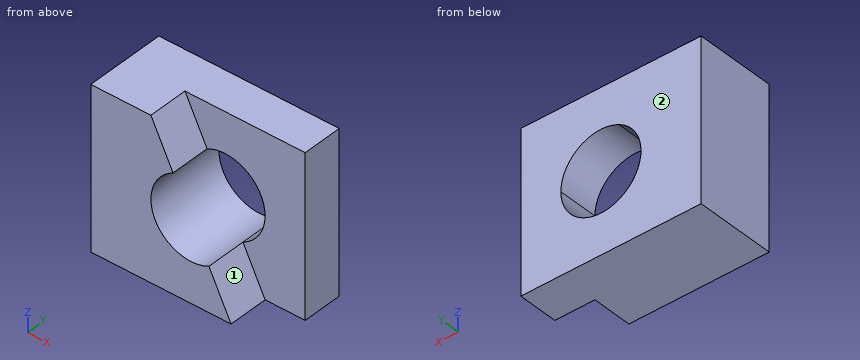
```python
from build123d import *

# Parameters (mm, degrees)
F0_W     = 57.15
F0_H     = 50.8
F1_DEPTH = 25.4
F3_DEPTH = 12.7
F5_DEPTH = 25.4


# Not quite as in the source:
# - a feature of the source that left no trace in its solid (it failed there, or was rolled back) is left out


with BuildPart() as f1:
    # F0 (on Front) → F1 (new body)
    with BuildSketch(Plane.XZ):
        with Locations((28.575, 25.4)):
            Rectangle(F0_W, F0_H)
    extrude(amount=F1_DEPTH)

    # F2 (on face) → F3 (cut)
    with BuildSketch(Plane.XZ.offset(25.4)):
        Polygon((44.45, 0), (57.15, 0), (57.15, 50.8), (19.05, 50.8), align=None)
    extrude(amount=-F3_DEPTH, mode=Mode.SUBTRACT)

    # F4 (on face) → F5 (cut)
    with BuildSketch(Plane.XZ.offset(25.4)):
        with BuildLine():
            ThreePointArc((37.4296126628, 14.0407746743), (42.5532652661, 18.7232148761), (44.45, 25.4))
            ThreePointArc((44.45, 25.4), (38.4267851239, 36.2032652661), (26.0703873372, 36.7592253257))
            Line((26.0703873372, 36.7592253257), (37.4296126628, 14.0407746743))
        make_face()
        with BuildLine():
            Line((37.4296126628, 14.0407746743), (26.0703873372, 36.7592253257))
            ThreePointArc((26.0703873372, 36.7592253257), (20.3907746743, 19.7203873372), (37.4296126628, 14.0407746743))
        make_face()
    extrude(amount=-F5_DEPTH, mode=Mode.SUBTRACT)


solid = f1.part
```
Work out the finished part from the listing and answer in its coordinate system (mm). Face numbers are marked on the shaded views. A direction names the side the tool comes from. Give positions to 0.01 mm unless a question says otherwise; leave off trailing zeros. Order: outer loops, then holes, each group sorted by start corner. A loop starts at its lowest first (then second) coordinate and runs counter-clockwise, first axis right, second up.
1. Straight lines are drawn through the part: L1, parallel to X at y = -1, z = 25; L2, parallel to Y at x = 47, z = 29.5; L3, parallel to X at y = -5.75, z = 32.5. For each, find the intervals that lie inside material, in ascending order.
Result sheet:
L1: x = 0 to 19.06, 44.44 to 57.15
L2: y = -12.7 to 0
L3: x = 0 to 21.22, 42.28 to 57.15
2. This flat-tipped pin is pushed along its axis until it touches: P1, Ø19, axis at x = 29, z = 16.5, coming from the -Y side. Where does it stop, or does it pass through?
Result sheet:
P1: stops at y = -25.4
3. Section B-B, the plane y = -6.5 is taken. Determine the outline of the cut face in (x, z), and give its area (3 significant figures).
Result sheet:
outline: (0, 0) - (57.15, 0) - (57.15, 50.8) - (0, 50.8) - close; hole circle Ø25.4 at (31.75, 25.4)
area: 2,400 mm2
4. Section A-A, the plane x = 31.75 is taken. Determine the outline of the cut face in (y, z).
Result sheet:
outline: (-25.4, 0) - (0, 0) - (0, 12.7) - (-25.4, 12.7) - close; (-12.7, 38.1) - (0, 38.1) - (0, 50.8) - (-12.7, 50.8) - close
5. Section D-D, the plane y = -19.75 is taken. Determine the outline of the cut face in (x, z).
Result sheet:
outline: (0, 0) - (44.45, 0) - (37.43, 14.04) arc R12.7 cw to (26.07, 36.76) - (19.05, 50.8) - (0, 50.8) - close
6. Section C-C, the plane z = 30 is taken. Determine the outline of the cut face in (x, y), and give its area (3 significant figures).
Result sheet:
outline: (0, -25.4) - (19.91, -25.4) - (19.91, 0) - (0, 0) - close; (43.59, -12.7) - (57.15, -12.7) - (57.15, 0) - (43.59, 0) - close
area: 678 mm2
7. For the marked faces 1 and 2, determine the directions among +Z, -Z, +X, -X, +Y, -Y from which every point of the face is accessible in a straight line to the end or side of a thin tool.
Result sheet:
face 1: +Z, +X, -Y
face 2: +Z, -Z, +X, -X, +Y
